from build123d import *

# Parameters (mm, degrees)
SKETCH1_W           = 39
SKETCH1_H           = 26
BOSS_EXTRUDE1_DEPTH = 2
SKETCH2_R           = 1.5
CUT_EXTRUDE1_DEPTH  = 24.521266973
SKETCH3_W           = 24.5
SKETCH3_H           = 16.5
BOSS_EXTRUDE2_DEPTH = 1
SKETCH4_W           = 15
SKETCH4_H           = 12
BOSS_EXTRUDE3_DEPTH = 3
SKETCH5_W           = 3.5
SKETCH5_H           = 3
BOSS_EXTRUDE4_DEPTH = 1
SKETCH6_R           = 1
BOSS_EXTRUDE5_DEPTH = 1
FILLET1_R           = 3


with BuildPart() as part:
    # Sketch1 → Boss-Extrude1 (new body)
    with BuildSketch(Plane(origin=(0, 0, 0), x_dir=(1, 0, 0), z_dir=(0, 1, 0))):
        Rectangle(SKETCH1_W, SKETCH1_H)
    extrude(amount=BOSS_EXTRUDE1_DEPTH)

    # Sketch2 → Cut-Extrude1 (cut, through all)
    with BuildSketch(Plane(origin=(0, 2, 0), x_dir=(1, 0, 0), z_dir=(0, 1, 0))):
        with Locations(Location((-16.5, 10, 0), (0, 0, 270))):
            Circle(SKETCH2_R)
        with Locations(Location((-16.5, -10, 0), (0, 0, 270))):
            Circle(SKETCH2_R)
        with Locations(Location((16.5, -10, 0), (0, 0, 270))):
            Circle(SKETCH2_R)
        with Locations(Location((16.5, 10, 0), (0, 0, 270))):
            Circle(SKETCH2_R)
    extrude(amount=-CUT_EXTRUDE1_DEPTH, mode=Mode.SUBTRACT)

    # Sketch3 → Boss-Extrude2 (add)
    with BuildSketch(Plane(origin=(0, 2, 0), x_dir=(1, 0, 0), z_dir=(0, 1, 0))):
        with Locations((7.75, 0)):
            Rectangle(SKETCH3_W, SKETCH3_H)
    extrude(amount=BOSS_EXTRUDE2_DEPTH)

    # Sketch4 → Boss-Extrude3 (add)
    with BuildSketch(Plane(origin=(0, 3, 0), x_dir=(1, 0, 0), z_dir=(0, 1, 0))):
        with Locations((5, 0)):
            Rectangle(SKETCH4_W, SKETCH4_H)
    extrude(amount=BOSS_EXTRUDE3_DEPTH)

    # Sketch5 → Boss-Extrude4 (add)
    with BuildSketch(Plane(origin=(0, 2, 0), x_dir=(1, 0, 0), z_dir=(0, 1, 0))):
        with Locations((-12.75, 3.5)):
            Rectangle(SKETCH5_W, SKETCH5_H)
        with Locations((-12.75, -4.5)):
            Rectangle(SKETCH5_W, SKETCH5_H)
    extrude(amount=BOSS_EXTRUDE4_DEPTH)

    # Sketch6 → Boss-Extrude5 (add)
    with BuildSketch(Plane(origin=(0, 3, 0), x_dir=(1, 0, 0), z_dir=(0, 1, 0))):
        with Locations(Location((-12.75, 3.5, 0), (0, 0, 270))):
            Circle(SKETCH6_R)
        with Locations(Location((-12.75, -4.5, 0), (0, 0, 270))):
            Circle(SKETCH6_R)
    extrude(amount=BOSS_EXTRUDE5_DEPTH)

    # Fillet1
    fillet1_edges = [part.edges().sort_by_distance(p)[0] for p in [
        (19.5, 1, 13),
        (-19.5, 1, 13),
        (-19.5, 1, -13),
        (19.5, 1, -13),
    ]]
    fillet(fillet1_edges, radius=FILLET1_R)


solid = part.part
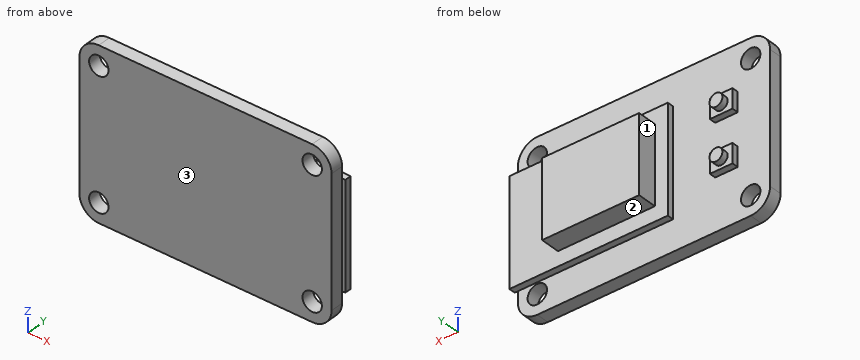
Verification items for the finished model (mm, model axes). Face numbers are marked on the shaded views. A direction names the side the tool comes from. Coordinates: 2 decimals unless noted, no trailing zeros. Order: outer loops, then holes, each group sorted by start corner. A loop starts at its lowest first (then second) coordinate and runs counter-clockwise, first axis right, second up. Notation, with made-up numbers: (45.25, 28) -> (87.25, 28) arc R15 cw to (87.25, 51) -> close; hole circle Ø11 at (30, 35). An arc over 180 degrees is marked (long way). Put each result on its own line as item: value. Start each with the question number.
1. Cross-section at A-A, the plane y = 2.6. Record the boundary of the cut face in (x, z).
2. Cross-section at D-D, the plane y = 0.65. Record the boundary of the cut face in (x, z), then the cut area to 3 significant figures.
3. Material ranges on L1, parallel to X at y = 1, z = -10; L2, parallel to X at y = 2.7, z = 5.25; L3, parallel to Z at x = 12, y = 2.9, recorded low to high. Write a range as [from, to].
4. Cross-section at C-C, the plane z = -11. Record the boundary of the cut face in (x, y), then the cut area to 3 significant figures.
5. Cross-section at B-B, the plane x = 3. Record the boundary of the cut face in (y, z).
6. Go/stop test with flat-tipped pins: pin 1 Ø0.8 at (y, z) = (2.5, 4.5) entering from -X; pin 2 Ø13 at (x, z) = (-5, -2) entering from +Y; pin 3 Ø1.5 at (x, y) = (7, 4.5) entering from +Z; pin 4 Ø2 at (x, z) = (-12.5, 5) entering from +Y. Record where each tip stops, or that it passes through.
7. Access from +Z, -Z, +X, -X, +Y, -Y to the whole of each face (thin tool, end or side, straight path). Record for the marked faces 1, 2 and 3.
Computed:
1. outline: (-14.5, -5) -> (-11, -5) -> (-11, -2) -> (-14.5, -2) -> close; (-14.5, 3) -> (-11, 3) -> (-11, 6) -> (-14.5, 6) -> close; (-4.5, -8.25) -> (20, -8.25) -> (20, 8.25) -> (-4.5, 8.25) -> close
2. outline: (-19.5, -10) arc R3 ccw to (-16.5, -13) -> (16.5, -13) arc R3 ccw to (19.5, -10) -> (19.5, 10) arc R3 ccw to (16.5, 13) -> (-16.5, 13) arc R3 ccw to (-19.5, 10) -> close; hole circle Ø3 at (-16.5, -10); hole circle Ø3 at (-16.5, 10); hole circle Ø3 at (16.5, -10); hole circle Ø3 at (16.5, 10)
2. area: 978 mm2
3. L1: [-19.5, -18], [-15, 15], [18, 19.5]
3. L2: [-14.5, -11], [-4.5, 20]
3. L3: [-8.25, 8.25]
4. outline: (-19.33, 0) -> (-17.62, 0) -> (-17.62, 2) -> (-19.33, 2) -> close; (-15.38, 0) -> (15.38, 0) -> (15.38, 2) -> (-15.38, 2) -> close; (17.62, 0) -> (19.33, 0) -> (19.33, 2) -> (17.62, 2) -> close
4. area: 68.4 mm2
5. outline: (0, -13) -> (2, -13) -> (2, -8.25) -> (3, -8.25) -> (3, -6) -> (6, -6) -> (6, 6) -> (3, 6) -> (3, 8.25) -> (2, 8.25) -> (2, 13) -> (0, 13) -> close
6. pin 1: x = -14.5
6. pin 2: y = 6
6. pin 3: z = 6
6. pin 4: y = 4
7. face 1: +Z, -Z, +Y
7. face 2: -Z, +X, -X, +Y
7. face 3: +Z, -Z, +X, -X, -Y
